Model file for the job. Use its own axes, mm. Give positions to 0.01 mm unless a question says otherwise; leave off trailing zeros. Order: outer loops, then holes, each group sorted by start corner. A loop starts at its lowest first (then second) coordinate and runs counter-clockwise, first axis right, second up. Notation, with made-up numbers: (-19, -31) - (11, -31) arc R17 cw to (11, -15) - close; hole circle Ø1 at (70.5, 60.25). An arc over 180 degrees is marked (long way). Return JSON: item names as keys, results as strings. Group by question number.
from build123d import *

# Parameters (mm, degrees)
SKETCH1_R           = 1.5
SKETCH1_R_2         = 5
SKETCH1_R_3         = 75
BOSS_EXTRUDE1_DEPTH = 5


with BuildPart() as part:
    # Sketch1 → Boss-Extrude1 (new body)
    with BuildSketch(Plane.XY):
        Polygon((-90, 145.000003033), (-90, 140.000003033), (-109, 140.000003033), (-109, 108.00000182), (-104, 108.00000182), (-104, 98.00000182), (-99.000966482, 98.00000182), (-99.000966482, 94.50000182), (-96.000966482, 94.50000182), (-96.000966482, 95.60000182), (-93.700966482, 95.60000182), (-93.700966482, 94.50000182), (-89.000966482, 94.50000182), (-89.000966482, 91.50000182), (-93.700966482, 91.50000182), (-93.700966482, 90.40000182), (-96.000966482, 90.40000182), (-96.000966482, 91.50000182), (-99.000966482, 91.50000182), (-99.000966482, 88.00000182), (-104, 88.00000182), (-104, 78.00000182), (-109, 78.00000182), (-109, 46.000000607), (-104, 46.000000607), (-104, 36.000000607), (-99.000966482, 36.000000607), (-99.000966482, 32.500000607), (-96.000966482, 32.500000607), (-96.000966482, 33.600000607), (-93.700966482, 33.600000607), (-93.700966482, 32.500000607), (-89.000966482, 32.500000607), (-89.000966482, 29.500000607), (-93.700966482, 29.500000607), (-93.700966482, 28.400000607), (-96.000966482, 28.400000607), (-96.000966482, 29.500000607), (-99.000966482, 29.500000607), (-99.000966482, 26.000000607), (-104, 26.000000607), (-104, 16.000000607), (-109, 16.000000607), (-109, -16.000000607), (-104, -16.000000607), (-104, -26.000000607), (-99.000966482, -26.000000607), (-99.000966482, -29.500000607), (-96.000966482, -29.500000607), (-96.000966482, -28.400000607), (-93.700966482, -28.400000607), (-93.700966482, -29.500000607), (-89.000966482, -29.500000607), (-89.000966482, -32.500000607), (-93.700966482, -32.500000607), (-93.700966482, -33.600000607), (-96.000966482, -33.600000607), (-96.000966482, -32.500000607), (-99.000966482, -32.500000607), (-99.000966482, -36.000000607), (-104, -36.000000607), (-104, -46.000000607), (-109, -46.000000607), (-109, -78.00000182), (-104, -78.00000182), (-104, -88.00000182), (-99.000966482, -88.00000182), (-99.000966482, -91.50000182), (-96.000966482, -91.50000182), (-96.000966482, -90.40000182), (-93.700966482, -90.40000182), (-93.700966482, -91.50000182), (-89.000966482, -91.50000182), (-89.000966482, -94.50000182), (-93.700966482, -94.50000182), (-93.700966482, -95.60000182), (-96.000966482, -95.60000182), (-96.000966482, -94.50000182), (-99.000966482, -94.50000182), (-99.000966482, -98.00000182), (-104, -98.00000182), (-104, -108.00000182), (-109, -108.00000182), (-109, -140.000003033), (-90, -140.000003033), (-90, -145.000003033), (-60, -145.000003033), (-60, -140.000003033), (-40, -140.000003033), (-40, -145.000003033), (-10, -145.000003033), (-10, -140.000003033), (10, -140.000003033), (10, -145.000003033), (40, -145.000003033), (40, -140.000003033), (60, -140.000003033), (60, -145.000003033), (90, -145.000003033), (90, -140.000003033), (109, -140.000003033), (109, -108.00000182), (104, -108.00000182), (104, -98.00000182), (99.000966482, -98.00000182), (99.000966482, -94.50000182), (96.000966482, -94.50000182), (96.000966482, -95.60000182), (93.700966482, -95.60000182), (93.700966482, -94.50000182), (89.000966482, -94.50000182), (89.000966482, -91.50000182), (93.700966482, -91.50000182), (93.700966482, -90.40000182), (96.000966482, -90.40000182), (96.000966482, -91.50000182), (99.000966482, -91.50000182), (99.000966482, -88.00000182), (104, -88.00000182), (104, -78.00000182), (109, -78.00000182), (109, -46.000000607), (104, -46.000000607), (104, -36.000000607), (99.000966482, -36.000000607), (99.000966482, -32.500000607), (96.000966482, -32.500000607), (96.000966482, -33.600000607), (93.700966482, -33.600000607), (93.700966482, -32.500000607), (89.000966482, -32.500000607), (89.000966482, -29.500000607), (93.700966482, -29.500000607), (93.700966482, -28.400000607), (96.000966482, -28.400000607), (96.000966482, -29.500000607), (99.000966482, -29.500000607), (99.000966482, -26.000000607), (104, -26.000000607), (104, -16.000000607), (109, -16.000000607), (109, 16.000000607), (104, 16.000000607), (104, 26.000000607), (99.000966482, 26.000000607), (99.000966482, 29.500000607), (96.000966482, 29.500000607), (96.000966482, 28.400000607), (93.700966482, 28.400000607), (93.700966482, 29.500000607), (89.000966482, 29.500000607), (89.000966482, 32.500000607), (93.700966482, 32.500000607), (93.700966482, 33.600000607), (96.000966482, 33.600000607), (96.000966482, 32.500000607), (99.000966482, 32.500000607), (99.000966482, 36.000000607), (104, 36.000000607), (104, 46.000000607), (109, 46.000000607), (109, 78.00000182), (104, 78.00000182), (104, 88.00000182), (99.000966482, 88.00000182), (99.000966482, 91.50000182), (96.000966482, 91.50000182), (96.000966482, 90.40000182), (93.700966482, 90.40000182), (93.700966482, 91.50000182), (89.000966482, 91.50000182), (89.000966482, 94.50000182), (93.700966482, 94.50000182), (93.700966482, 95.60000182), (96.000966482, 95.60000182), (96.000966482, 94.50000182), (99.000966482, 94.50000182), (99.000966482, 98.00000182), (104, 98.00000182), (104, 108.00000182), (109, 108.00000182), (109, 140.000003033), (90, 140.000003033), (90, 145.000003033), (60, 145.000003033), (60, 140.000003033), (40, 140.000003033), (40, 145.000003033), (10, 145.000003033), (10, 140.000003033), (-10, 140.000003033), (-10, 145.000003033), (-40, 145.000003033), (-40, 140.000003033), (-60, 140.000003033), (-60, 145.000003033), align=None)
        with Locations((-75, -142.500003033)):
            Circle(SKETCH1_R, mode=Mode.SUBTRACT)
        with Locations((-25, -142.500003033)):
            Circle(SKETCH1_R, mode=Mode.SUBTRACT)
        with Locations((25, -142.500003033)):
            Circle(SKETCH1_R, mode=Mode.SUBTRACT)
        with Locations((0, -108.739893094)):
            Circle(SKETCH1_R_2, mode=Mode.SUBTRACT)
        with Locations((75, -142.500003033)):
            Circle(SKETCH1_R, mode=Mode.SUBTRACT)
        with Locations((-75, 142.500003033)):
            Circle(SKETCH1_R, mode=Mode.SUBTRACT)
        with Locations((-25, 142.500003033)):
            Circle(SKETCH1_R, mode=Mode.SUBTRACT)
        Circle(SKETCH1_R_3, mode=Mode.SUBTRACT)
        with Locations((25, 142.500003033)):
            Circle(SKETCH1_R, mode=Mode.SUBTRACT)
        with Locations((75, 142.500003033)):
            Circle(SKETCH1_R, mode=Mode.SUBTRACT)
    extrude(amount=BOSS_EXTRUDE1_DEPTH)


solid = part.part
(1) Slice it at B-B (x = 0). Give the cut face in (y, z).
(2) Drill centre lines: L1, parallel to Y at x = -91.5, z = 3.7; L2, parallel to Y at x = -15, z = 4.35; L3, parallel to X at y = -91, z = 2.45. Where is each one in solid material? Low to high.
(3) Slice it at C-C (x = -69). Give the cut face in (y, z), and give its area (3 significant figures).
(4) Slice it at D-D (y = 103.5). Give the cut face in (x, z).
(5) Drop flat-ended pins along their axis: pin 1 Ø0.9 at (y, z) = (29, 3.5) entering from -X; pin 2 Ø2.5 at (x, z) = (97, 2) entering from -Y; pin 3 Ø1.5 at (y, z) = (82.5, 1.5) entering from -X; pin 4 Ø8 at (x, y) = (6.5, 104) entering from -Z. Give the stop position or say it passes through.
(6) Pull direction Y, two halves, no side cores. Call faces 1 (the face through (-74, 34, 5)), 2 (the face through (-1.08, -113.62, 2.46)), 3 (the face through (-9.764, 74.362, 2.465)): released by +Y, released by -Y, zero draft, split by the parting line, or undercut.
(7) Slice it at A-A (y = 0). Give the cut face in (x, z).
Result set:
{
 "1": {"outline": "(-140, 0) - (-113.74, 0) - (-113.74, 5) - (-140, 5) - close; (-103.74, 0) - (-75, 0) - (-75, 5) - (-103.74, 5) - close; (75, 0) - (140, 0) - (140, 5) - (75, 5) - close"},
 "2": {"L1": "y = -140 to -94.5, -91.5 to -32.5, -29.5 to 29.5, 32.5 to 91.5, 94.5 to 140", "L2": "y = -145 to -73.48, 73.48 to 145", "L3": "x = -99 to -96, -93.7 to 93.7, 96 to 99"},
 "3": {"outline": "(-145, 0) - (-29.39, 0) - (-29.39, 5) - (-145, 5) - close; (29.39, 0) - (145, 0) - (145, 5) - (29.39, 5) - close", "area": "1,160 mm²"},
 "4": {"outline": "(-104, 0) - (104, 0) - (104, 5) - (-104, 5) - close"},
 "5": {"pin 1": "stops at x = -99", "pin 2": "stops at y = -140", "pin 3": "stops at x = -104", "pin 4": "stops at z = 0"},
 "6": {"face 1": "zero draft", "face 2": "undercut", "face 3": "undercut"},
 "7": {"outline": "(-109, 0) - (-75, 0) - (-75, 5) - (-109, 5) - close; (75, 0) - (109, 0) - (109, 5) - (75, 5) - close"}
}
